Build history of the part. All positions in model axes, mm. A direction names the side the tool comes from. Round coordinates to 2 decimals unless told otherwise and drop trailing zeros. Write each loop counter-clockwise with the first axis right and the second up, starting at its lowest first coordinate (ties: lowest second). Pieces come first, ordered by that corner, then holes. Notation, with made-up numbers: M 59,21 L 73,21 A5 ccw 73,25 Z; hole C 81,12.25 d1. An arc over 180 degrees is marked long. Write item = value, one per line.
from build123d import *

# Parameters (mm, degrees)
F2_R     = 5.715
F3_DEPTH = 25.4
F4_R     = 3.175
F5_DEPTH = 38.1


with BuildPart() as f1:
    # F0 (on Front) → F1 (revolve)
    with BuildSketch(Plane.XZ):
        Polygon((10.795, 42.584405), (0, 42.584405), (0, 29.884405), (5.715, 29.884405), align=None)
    revolve(axis=Axis((0, 0, 36.234405), (0, 0, -1)))

    # F2 (on face) → F3 (join)
    with BuildSketch(Plane(origin=(0, 0, 29.884405), x_dir=(1, 0, 0), z_dir=(0, 0, -1))):
        Circle(F2_R)
    extrude(amount=F3_DEPTH)

    # F4 (on face) → F5 (cut)
    with BuildSketch(Plane.XY.offset(42.584405)):
        Circle(F4_R)
    extrude(amount=-F5_DEPTH, mode=Mode.SUBTRACT)


solid = f1.part
1. Band-saw the part on C-C (z = 19). List the corners of the cut face in (x, y) (3 decimals), plus the area to 3 significant figures.
Responses:
outline = C 0,0 d11.43; hole C 0,0 d6.35
area = 70.9 mm²
2. Tool access for faces 1 (the face through (-3, 2, 42.584)), 2 (the face through (5.45, -1.72, 17.36)): list every direction of +Z, -Z, +X, -X, +Y, -Y with a clear straight run to the whole face (end or side of a thin tool).
Responses:
face_1 = +Z, +X, -X, +Y, -Y
face_2 = -Z
3. Band-saw the part on A-A (x = 0). List the corners of the cut face in (y, z) (3 decimals), plus the area to 3 significant figures.
Responses:
outline = M -10.795,42.584 L -5.715,29.884 L -5.715,4.484 L -3.175,4.484 L -3.175,42.584 Z; M 3.175,4.484 L 5.715,4.484 L 5.715,29.884 L 10.795,42.584 L 3.175,42.584 Z
area = 258 mm²
4. Flat gauge pins, fed straight in: pin 1 (4 mm diameter, centred on y = -4.5, z = 24, fed in from -X); pin 2 (10 mm diameter, centred on y = -7, z = 35, fed in from -X); pin 3 (3 mm diameter, centred on y = -6, z = 28.5, fed in from -X). Where does each tip first touch, or does it go through?
Responses:
pin_1 = -5.14
pin_2 = -8.5
pin_3 = -3.52
5. Probe probe 1 along Y at (x, z) = (0, 21) (3 decimals); probe 2 along Y at (x, z) = (2, 21.5); probe 3 along X at (y, z) = (-0.5, 11). List the from-to ranges inside material, lowest first.
Responses:
probe_1 = -5.715 to -3.175, 3.175 to 5.715
probe_2 = -5.35 to -2.47, 2.47 to 5.35
probe_3 = -5.69 to -3.14, 3.14 to 5.69
